Input: part model. Units: mm. Frame: model coordinates. Round coordinates to 2 decimals unless told otherwise and drop trailing zeros. Loops run counter-clockwise (first coordinate to the right, second up) from the corner with the lowest first, then second, coordinate; pieces in that order, holes last. Notation, with made-up numbers: M 68.5,20.25 L 118.5,20.25 A14 cw 118.5,33.25 Z; hole C -25.75,44.5 d9. An arc over 180 degrees is marked long. Return JSON: item names as keys, results as strings. Group by question number.
1) Section A-A (y = -1.5). Output: boundary loops of the cut face in (x, z).
2) Material intervals for line 1 (Y direction, x = -23.5, z = -0.15); line 2 (Y direction, x = -8, z = 2.1); line 3 (Z direction, x = -21, y = -0.75), sorted ascending. Write a range as from..to.
3) Section C-C (z = 0). Output: boundary loops of the cut face in (x, y), plus the area to 3 significant figures.
4) Contact query for a flat-ended pin moving along its axis: P1, Ø1, axis at y = -1, z = -1.5, coming from the -X side. Output: stop coordinate, or through.
5) Section B-B (x = -18.5). Output: boundary loops of the cut face in (y, z), plus the area to 3 significant figures.
from build123d import *

# Parameters (mm, degrees)
SKETCH_2_W         = 65
SKETCH_2_H         = 2.5
DOME_3_FACE_RADIUS = 2.5
DOME_3_HEIGHT      = 2.5
DOME_4_FACE_RADIUS = 2.5
DOME_4_HEIGHT      = 2.5


with BuildPart() as part:
    # 草圖2 → 旋轉2 (revolve)
    with BuildSketch(Plane.XY):
        with Locations((3.5, 1.25)):
            Rectangle(SKETCH_2_W, SKETCH_2_H)
    revolve(axis=Axis((-29, 0, 0), (1, 0, 0)))

    # 圓頂3: a dome of height H over a round flat face of radius A is a cap of a sphere of radius (A * A + H * H) / (2 * H)
    dome_3_r = (DOME_3_FACE_RADIUS * DOME_3_FACE_RADIUS + DOME_3_HEIGHT * DOME_3_HEIGHT) / (2 * DOME_3_HEIGHT)
    dome_3_base = Plane((36, 0, 0), z_dir=(1, 0, 0))
    with Locations(dome_3_base.offset(DOME_3_HEIGHT - dome_3_r)):
        dome_3_ball = Sphere(dome_3_r, mode=Mode.PRIVATE)
    add(split(dome_3_ball, bisect_by=dome_3_base, keep=Keep.TOP, mode=Mode.PRIVATE))

    # 圓頂4: a dome of height H over a round flat face of radius A is a cap of a sphere of radius (A * A + H * H) / (2 * H)
    dome_4_r = (DOME_4_FACE_RADIUS * DOME_4_FACE_RADIUS + DOME_4_HEIGHT * DOME_4_HEIGHT) / (2 * DOME_4_HEIGHT)
    dome_4_base = Plane((-29, 0, 0), z_dir=(-1, 0, 0))
    with Locations(dome_4_base.offset(DOME_4_HEIGHT - dome_4_r)):
        dome_4_ball = Sphere(dome_4_r, mode=Mode.PRIVATE)
    add(split(dome_4_ball, bisect_by=dome_4_base, keep=Keep.TOP, mode=Mode.PRIVATE))


solid = part.part
Returned:
{
 "1": {"outline": "M -29,-2 L 36,-2 A2 ccw 36,2 L -29,2 A2 ccw Z"},
 "2": {"line 1": "y = -2.5..2.5", "line 2": "y = -1.36..1.36", "line 3": "z = -2.38..2.38"},
 "3": {"outline": "M -29,-2.5 L 36,-2.5 A2.5 ccw 36,2.5 L -29,2.5 A2.5 ccw Z", "area": "345 mm^2"},
 "4": {"P1": "stops at x = -31.13"},
 "5": {"outline": "C 0,0 d5", "area": "19.6 mm^2"}
}
